from build123d import *

# Parameters (mm, degrees)
SKETCH6_W           = 25.262112462
SKETCH6_H           = 25.4
BOSS_EXTRUDE3_DEPTH = 127
SKETCH8_R           = 6.263004549
CUT_EXTRUDE1_DEPTH  = 25.4
SKETCH9_W           = 21.756912462
SKETCH9_H           = 21.8948
CUT_EXTRUDE2_DEPTH  = 127


with BuildPart() as part:
    # Sketch6 → Boss-Extrude3 (new body)
    with BuildSketch(Plane(origin=(0, 0, 0), x_dir=(1, 0, 0), z_dir=(0, 1, 0))):
        with Locations((12.631056231, 12.7)):
            Rectangle(SKETCH6_W, SKETCH6_H)
    extrude(amount=BOSS_EXTRUDE3_DEPTH)

    # Sketch8 → Cut-Extrude1 (cut)
    with BuildSketch(Plane.XY):
        with Locations((11.587222139, 119.780054764)):
            Circle(SKETCH8_R)
    extrude(amount=-CUT_EXTRUDE1_DEPTH, mode=Mode.SUBTRACT)

    # Sketch9 → Cut-Extrude2 (cut)
    with BuildSketch(Plane(origin=(0, 0, 0), x_dir=(-1, 0, 0), z_dir=(0, -1, 0))):
        with Locations((-12.631056231, 12.7)):
            Rectangle(SKETCH9_W, SKETCH9_H)
    extrude(amount=-CUT_EXTRUDE2_DEPTH, mode=Mode.SUBTRACT)


solid = part.part
Read the model definition and answer for the solid it produces. Units are mm, in the model's axes. A direction names the side the tool comes from. Coordinates: 2 decimals unless noted, no trailing zeros. Write each loop counter-clockwise with the first axis right and the second up, starting at its lowest first coordinate (ties: lowest second). Pieces come first, ordered by that corner, then holes. Notation, with made-up numbers: M 40.5,69.25 L 90.5,69.25 A18 cw 90.5,97.25 Z; hole C -32.75,-10 d5. An arc over 180 degrees is marked long. Use a Markdown table: item, result.
Q1. Which of the six approach directions +Z, -Z, +X, -X, +Y, -Y give full straight-line access (tool end or side, diameter ignored) to faces 4 (the face through (10.77, 125.99, -24.51)), 5 (the face through (23.51, 63, -13))?
Answer block:
| item | result |
|---|---|
| face 4 | +Z, -Z |
| face 5 | +Y, -Y |
Q2. The part is cut by section A-A, the plane y = 62. Write down the section's boundary in (x, z).
Answer block:
| item | result |
|---|---|
| outline | M 0,-25.4 L 25.26,-25.4 L 25.26,0 L 0,0 Z; hole M 1.75,-23.65 L 23.51,-23.65 L 23.51,-1.75 L 1.75,-1.75 Z |
Q3. The part is cut by section B-B, the plane x = 21.5. Write down the section's boundary in (y, z).
Answer block:
| item | result |
|---|---|
| outline | M 0,-25.4 L 127,-25.4 L 127,-23.65 L 0,-23.65 Z; M 0,-1.75 L 127,-1.75 L 127,0 L 0,0 Z |
Q4. Straight lines are drawn through the part: L1, parallel to X at y = 6.5, z = -15; L2, parallel to Z at x = 15.25, y = 55. For each, find the intervals that lie inside material, in ascending order. Write a range as [from, to].
Answer block:
| item | result |
|---|---|
| L1 | x = [0, 1.75], [23.51, 25.26] |
| L2 | z = [-25.4, -23.65], [-1.75, 0] |
Q5. Determine the mould class of faces 1 (the face through (1, 127, -13)), 2 (the face through (13, 63, -23.647)), 3 (the face through (12, 63, 0)) for opening direction Z: released by +Z, released by -Z, zero draft, split by the parting line, or undercut.
Answer block:
| item | result |
|---|---|
| face 1 | zero draft |
| face 2 | undercut |
| face 3 | released by +Z |
Q6. The part is cut by section C-C, the plane z = -7.75. Write down the section's boundary in (x, y), then the cut area to 3 significant figures.
Answer block:
| item | result |
|---|---|
| outline | M 0,0 L 1.75,0 L 1.75,127 L 0,127 Z; M 23.51,0 L 25.26,0 L 25.26,127 L 23.51,127 Z |
| area | 445 mm2 |
Q7. The part is cut by section D-D, the plane x = 12.5. Write down the section's boundary in (y, z).
Answer block:
| item | result |
|---|---|
| outline | M 0,-25.4 L 113.58,-25.4 L 113.58,-23.65 L 0,-23.65 Z; M 0,-1.75 L 113.58,-1.75 L 113.58,0 L 0,0 Z; M 125.98,-25.4 L 127,-25.4 L 127,-23.65 L 125.98,-23.65 Z; M 125.98,-1.75 L 127,-1.75 L 127,0 L 125.98,0 Z |
